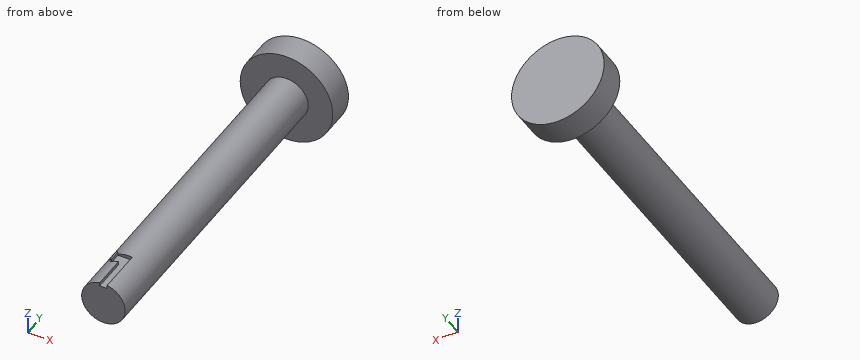
```python
from build123d import *

# Parameters (mm, degrees)
F0_R      = 2.9845
F1_DEPTH  = 44.45
F3_R      = 6.35
F4_DEPTH  = 3.81
F5_W      = 1.016
F5_H      = 1.016
F6_DEPTH  = 25.4
F8_DEPTH  = 1.524
F9_W      = 0.2032
F9_H      = 1.524
F10_DEPTH = 0.4572
F11_DEPTH = 19.304


with BuildPart() as f1:
    # F0 (on Front) → F1 (new body)
    with BuildSketch(Plane.XZ):
        Circle(F0_R)
    extrude(amount=F1_DEPTH)

    # F3 (on face) → F4 (join)
    with BuildSketch(Plane(origin=(0, 0, 0), x_dir=(-1, 0, 0), z_dir=(0, 1, 0))):
        Circle(F3_R)
    extrude(amount=F4_DEPTH)

    # F5 (on face) → F6 (cut)
    with BuildSketch(Plane.XZ.offset(44.45)):
        with Locations((0, 2.9843547381)):
            Rectangle(F5_W, F5_H)
    extrude(amount=-F6_DEPTH, mode=Mode.SUBTRACT)

    # F7 (on face) → F8 (cut)
    with BuildSketch(Plane.YZ.offset(-0.508)):
        Polygon((-39.878, 2.9409481889), (-39.878, 2.7086514635), (-39.878, 2.4763547381), (-38.354, 2.4763547381), (-38.354, 2.9409481889), align=None)
    extrude(amount=-F8_DEPTH, mode=Mode.SUBTRACT)

    # F9 (on face) → F10 (join)
    with BuildSketch(Plane.XY.offset(2.4763547381)):
        with Locations((-1.564205349, -39.116)):
            Rectangle(F9_W, F9_H)
    extrude(amount=F10_DEPTH)

    # F11 (add): a face of the model
    f11_faces = [f1.faces().sort_by_distance(p)[0] for p in [
        (0, -19.05, 2.7233604539),
    ]]
    extrude(f11_faces, amount=F11_DEPTH)


solid = f1.part
```
Design review of the part built by this model. Coordinates are the model's own, in mm. Give positions to 0.01 mm unless a question says otherwise; leave off trailing zeros. Loops run counter-clockwise (first coordinate to the right, second up) from the corner with the lowest first, then second, coordinate; pieces in that order, holes last. Notation, with made-up numbers: M -37.5,14.25 L -29.5,14.25 A21 cw -29.5,41.25 Z; hole C 1,80.5 d3. An arc over 180 degrees is marked long. Return JSON: item names as keys, results as strings. Group by question number.
Item 1: Insertion check: pin 1 Ø3 at (x, z) = (-2.5, -4) entering from -Y; pin 2 Ø4 at (x, y) = (-3.5, -20) entering from +Z; pin 3 Ø5 at (y, z) = (-21, -2.5) entering from +X; pin 4 Ø6 at (x, z) = (-4.5, 3.5) entering from -Y. Each pin has a flat end and moves straight along its axis. Give the tip position at first contact, or say it passes through.
Item 2: For probe 1 along Y at (x, z) = (-3, -0.5); probe 2 along Z at (x, y) = (-1.5, -11); probe 3 along X at (y, z) = (-27, -1.25), list the stretches that pass through material, from the lowest coordinate up.
Item 3: We need section C-C (y = -36). Give the boundary of the cut face in (x, z), and give its area (3 significant figures).
Item 4: We need section D-D (x = -2.25). Give the boundary of the cut face in (y, z), and give its area (3 significant figures).
Item 5: We need section A-A (z = 0). Give the boundary of the cut face in (x, y).
Item 6: We need section B-B (x = 0). Give the boundary of the cut face in (y, z).
Output:
{
 "1": {"pin 1": "stops at y = 0", "pin 2": "stops at z = 2.58", "pin 3": "stops at x = 2.98", "pin 4": "stops at y = -44.45"},
 "2": {"probe 1": "y = 0 to 3.81", "probe 2": "z = -2.58 to 2.58", "probe 3": "x = -2.71 to 2.71"},
 "3": {"outline": "C 0,0 d5.97", "area": "28.0 mm^2"},
 "4": {"outline": "M -44.45,-1.96 L 0,-1.96 L 0,-5.94 L 3.81,-5.94 L 3.81,5.94 L 0,5.94 L 0,1.96 L -44.45,1.96 Z", "area": "220 mm^2"},
 "5": {"outline": "M -6.35,0 L -2.98,0 L -2.98,-44.45 L 2.98,-44.45 L 2.98,0 L 6.35,0 L 6.35,3.81 L -6.35,3.81 Z"},
 "6": {"outline": "M -44.45,-2.98 L 0,-2.98 L 0,-6.35 L 3.81,-6.35 L 3.81,6.35 L 0,6.35 L 0,2.98 L -38.35,2.98 L -38.35,2.48 L -44.45,2.48 Z"}
}
